```python
from build123d import *

# Parameters (mm, degrees)
F0_R     = 285.75
F0_R_2   = 284.0482
F1_DEPTH = 914.4
F2_W     = 381
F2_H     = 76.2
F3_DEPTH = 285.751


with BuildPart() as f1:
    # F0 (on Top) → F1 (new body)
    with BuildSketch(Plane.XY):
        Circle(F0_R)
        Circle(F0_R_2, mode=Mode.SUBTRACT)
    extrude(amount=F1_DEPTH)

    # F2 (on Front) → F3 (cut, through all)
    with BuildSketch(Plane.XZ):
        with Locations((0, 825.5)):
            Rectangle(F2_W, F2_H)
    extrude(amount=F3_DEPTH, mode=Mode.SUBTRACT)


solid = f1.part
```
Design review of the part built by this model. Coordinates are the model's own, in mm. Coordinates: 2 decimals unless noted, no trailing zeros. Loops run counter-clockwise (first coordinate to the right, second up) from the corner with the lowest first, then second, coordinate; pieces in that order, holes last. Notation, with made-up numbers: (53, -12.75) -> (95, -12.75) arc R30 ccw to (95, 9.25) -> close; hole circle Ø7 at (35.25, 32). An arc over 180 degrees is marked (long way). Answer as a JSON object with one key per item and string values.
Q1. Take a section at B-B on x = 0. Give the boundary of the cut face in (y, z), plus the area to 3 significant figures.
Answer block:
{"outline": "(-285.75, 0) -> (-284.05, 0) -> (-284.05, 787.4) -> (-285.75, 787.4) -> close; (-285.75, 863.6) -> (-284.05, 863.6) -> (-284.05, 914.4) -> (-285.75, 914.4) -> close; (284.05, 0) -> (285.75, 0) -> (285.75, 914.4) -> (284.05, 914.4) -> close", "area": "2,980 mm^2"}
Q2. Take a section at A-A on y = 0. Give the boundary of the cut face in (x, z), plus the area to 3 significant figures.
Answer block:
{"outline": "(-285.75, 0) -> (-284.05, 0) -> (-284.05, 914.4) -> (-285.75, 914.4) -> close; (284.05, 0) -> (285.75, 0) -> (285.75, 914.4) -> (284.05, 914.4) -> close", "area": "3,110 mm^2"}
Q3. Clearance check with flat-ended pins moving along their axes: pin 1 Ø6 at (x, z) = (-57, 248) entering from +Y; pin 2 Ø1 at (y, z) = (-70, 596.5) entering from -X; pin 3 Ø1.1 at (y, z) = (-212, 843.5) entering from +X. State where each tip first meets the part, or that it passes through.
Answer block:
{"pin 1": "stops at y = 280.6", "pin 2": "stops at x = -277.17", "pin 3": "stops at x = 192.2"}
Q4. To check wall thickness, follow L1, parallel to Y at x = 0, z = 500; L2, parallel to X at y = -33, z = 749; L3, parallel to X at y = 164.5, z = 844. State the ranges of each line that lie inside material, in increasing order.
Answer block:
{"L1": "y = -285.75 to -284.05, 284.05 to 285.75", "L2": "x = -283.84 to -282.12, 282.12 to 283.84", "L3": "x = -233.65 to -231.57, 231.57 to 233.65"}
Q5. The part is to be moulded in two halves that separate along Z. For faces 1 (the flat face through (13, -284, 863.6)), 2 (the flat face through (13, -284, 787.4)), say which applies: +Z half, -Z half, draft (parallel to the pull), parting line (faces both ways), or undercut.
Answer block:
{"face 1": "undercut", "face 2": "undercut"}
Q6. Take a section at D-D on z = 573. Give the boundary of the cut face in (x, y).
Answer block:
{"outline": "circle Ø571.5 at (0, 0); hole circle Ø568.1 at (0, 0)"}
